from build123d import *

# Parameters (mm, degrees)
F0_R            = 50.8
F1_DEPTH        = 25.4
F2_R            = 3.175
F3_DEPTH        = 25.401
F3_COPIES_COUNT = 6


# Not quite as in the source:
# - a pattern or mirror of a feature is missing from the dataset's text; its kind, count and spacing are read off the source's solid


with BuildPart() as f1:
    # F0 (on Top) → F1 (new body)
    with BuildSketch(Plane.XY):
        Circle(F0_R)
    extrude(amount=F1_DEPTH)

    # F2 (on face) → F3 (cut, through all)
    with BuildSketch(Plane.XY.offset(25.4)):
        with Locations((0, -31.75)):
            Circle(F2_R)
    f3 = extrude(amount=-F3_DEPTH, mode=Mode.SUBTRACT)

    # F3_copies: F3 ×6 about axis
    f3_copies_axis = Axis((0, 0, 0), (0, 0, 1))
    for i in range(1, F3_COPIES_COUNT):
        add(f3.rotate(f3_copies_axis, i * 360 / F3_COPIES_COUNT), mode=Mode.SUBTRACT)


solid = f1.part
For this review, take the finished solid that the model builds, in its own axes (mm). Give positions to 0.01 mm unless a question says otherwise; leave off trailing zeros. Loops run counter-clockwise (first coordinate to the right, second up) from the corner with the lowest first, then second, coordinate; pieces in that order, holes last.
Item 1: Take a section at C-C, the plane y = 31.75. State the section outline as (x, z) points (3 decimals), and give its area (3 significant figures).
Item 2: Draft analysis for pull direction Y (two halves, no side actions). For faces 1 (the flat face through (-1, 1, 25.4)), 2 (the cylindrical face through (24.563, -14.659, 12.878)), 3 (the cylindrical face through (24.324, 16.015, 12.878)), 4 (the cylindrical face through (-11.012, -49.592, 12.522)), state which applies: +Y half, -Y half, draft (parallel to the pull), parting line (faces both ways), or undercut.
Item 3: For line 1 along Y through (x, z) = (0, 5.25) (3 decimals); line 2 along X through (y, z) = (-15.5, 12); line 3 along Y through (x, z) = (-26.5, 4.5), list the stretches that pass through material, from the lowest coordinate up.
Item 4: Take a section at B-B, the plane z = 17. State the section outline as (x, y) points (3 decimals).
Item 5: Take a section at A-A, the plane x = 0. State the section outline as (y, z) points (3 decimals).
Item 6: Take a section at D-D, the plane x = 12. State the section outline as (y, z) points.
Item 7: Insertion check: pin 1 (5 mm diameter, centred on x = 24.5, z = 13, fed in from +Y); pin 2 (2 mm diameter, centred on x = 37.5, z = 12.5, fed in from +Y); pin 3 (5 mm diameter, centred on y = 25, z = 12.5, fed in from -X); pin 4 (5.5 mm diameter, centred on x = -27.5, y = 15.88, fed in from -Z). Each pin has a flat end and moves straight along its axis. Give the tip position at first contact, or say it passes through.
Calculated:
1. outline: (-39.656, 0) - (-3.175, 0) - (-3.175, 25.4) - (-39.656, 25.4) - close; (3.175, 0) - (39.656, 0) - (39.656, 25.4) - (3.175, 25.4) - close
1. area: 1,850 mm2
2. face 1: draft
2. face 2: undercut
2. face 3: undercut
2. face 4: parting line
3. line 1: y = -50.8 to -34.925, -28.575 to 28.575, 34.925 to 50.8
3. line 2: x = -48.38 to -30.65, -24.34 to 24.34, 30.65 to 48.38
3. line 3: y = -43.34 to -18.89, -12.86 to 12.86, 18.89 to 43.34
4. outline: circle Ø101.6 at (0, 0); hole circle Ø6.35 at (-27.496, -15.875); hole circle Ø6.35 at (-27.496, 15.875); hole circle Ø6.35 at (0, -31.75); hole circle Ø6.35 at (0, 31.75); hole circle Ø6.35 at (27.496, -15.875); hole circle Ø6.35 at (27.496, 15.875)
5. outline: (-50.8, 0) - (-34.925, 0) - (-34.925, 25.4) - (-50.8, 25.4) - close; (-28.575, 0) - (28.575, 0) - (28.575, 25.4) - (-28.575, 25.4) - close; (34.925, 0) - (50.8, 0) - (50.8, 25.4) - (34.925, 25.4) - close
6. outline: (-49.36, 0) - (49.36, 0) - (49.36, 25.4) - (-49.36, 25.4) - close
7. pin 1: stops at y = 45.79
7. pin 2: stops at y = 35.33
7. pin 3: stops at x = -45.55
7. pin 4: passes through
